Check sheet for the modelled part. Datum: model origin and axes. Units: mm. Coordinates: 2 decimals unless noted, no trailing zeros. Write each loop counter-clockwise with the first axis right and the second up, starting at its lowest first coordinate (ties: lowest second). Pieces come first, ordered by that corner, then holes. Notation, with made-up numbers: M -9,-14.5 L 40,-14.5 A27 ccw 40,4.5 Z; hole C 60.25,-13.75 d8. An arc over 180 degrees is marked long. Answer as CSV lines item,"result".
Autodesk Inventor part; units mm, degrees
ref_plane "YZ Plane" through (0, 0, 0) normal (1, 0, 0) x (0, 1, 0)
ref_plane "XZ Plane" through (0, 0, 0) normal (0, 1, 0) x (-1, 0, 0)
ref_plane "XY Plane" through (0, 0, 0) normal (0, 0, 1) x (1, 0, 0)
sketch "Sketch1" plane through (0, 0, 0) normal (0, 1, 0) x (-1, 0, 0)
  line L0 (-5, 10) -> (5, 10)
  line L1 (5, 10) -> (5, -10)
  line L2 (5, -10) -> (-5, -10)
  line L3 (-5, -10) -> (-5, 10)
  line L4 (-5, 10) -> (5, -10) construction
  line L5 (5, 10) -> (-5, -10) construction
  line L6 (12.5, 20) -> (-12.5, 20)
  line L7 (-12.5, 20) -> (-12.5, -110)
  line L8 (-12.5, -110) -> (12.5, -110)
  line L9 (12.5, -110) -> (12.5, 20)
  line L10 (1.59, -105) -> (-1.59, -105)
  line L11 (-1.59, -105) -> (-1.59, -90)
  line L12 (-1.59, -90) -> (1.59, -90)
  line L13 (1.59, -90) -> (1.59, -105)
  line L14 (1.59, -105) -> (-1.59, -90) construction
  line L15 (-1.59, -105) -> (1.59, -90) construction
  line L16 (7.5, -95.91) -> (-7.5, -95.91)
  line L17 (-7.5, -95.91) -> (-7.5, -99.09)
  line L18 (-7.5, -99.09) -> (7.5, -99.09)
  line L19 (7.5, -99.09) -> (7.5, -95.91)
  line L20 (7.5, -95.91) -> (-7.5, -99.09) construction
  line L21 (-7.5, -95.91) -> (7.5, -99.09) construction
  point P0 (0, 0)
  point P1 (0, 0)
  point P2 (0, 0)
  point P3 (0, -97.5)
  dimension "d24" = 10
  dimension "d25" = 20
  dimension "d26" = 25
  dimension "d27" = 130
  dimension "d28" = 20
  dimension "d29" = 12.5
  dimension "d37" = 3.18
  dimension "d38" = 15
  dimension "d39" = 15
  dimension "d40" = 3.18
  dimension "d41" = 12.5
  dimension "d42" = 12.5
extrude "Extrusion3" add sketch "Sketch1" along normal blind 3.18
properties part number "Brazo_Superior"
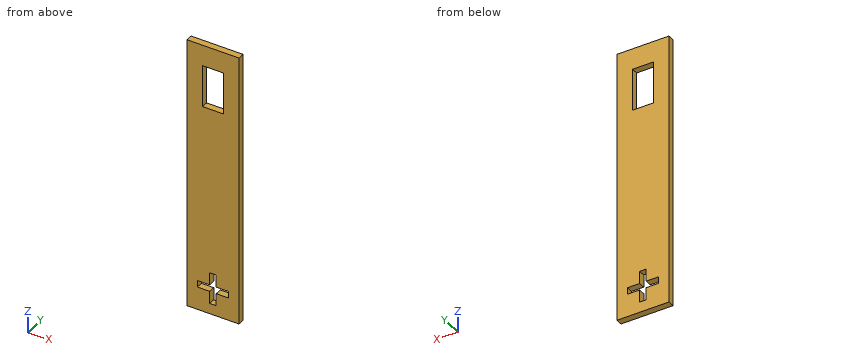
1) Section check B-B, the plane x = -0.25. Record the boundary of the cut face in (y, z), plus the area to 3 significant figures.
Answer key:
outline,"M 0,-110 L 3.18,-110 L 3.18,-105 L 0,-105 Z; M 0,-90 L 3.18,-90 L 3.18,-10 L 0,-10 Z; M 0,10 L 3.18,10 L 3.18,20 L 0,20 Z"
area,"302 mm2"
2) Section check A-A, the plane z = -97. Record the boundary of the cut face in (x, y).
Answer key:
outline,"M -12.5,0 L -7.5,0 L -7.5,3.18 L -12.5,3.18 Z; M 7.5,0 L 12.5,0 L 12.5,3.18 L 7.5,3.18 Z"
3) Section check C-C, the plane y = 0.75. Record the boundary of the cut face in (x, z), plus the area to 3 significant figures.
Answer key:
outline,"M -12.5,-110 L 12.5,-110 L 12.5,20 L -12.5,20 Z; hole M -7.5,-99.09 L -1.59,-99.09 L -1.59,-105 L 1.59,-105 L 1.59,-99.09 L 7.5,-99.09 L 7.5,-95.91 L 1.59,-95.91 L 1.59,-90 L -1.59,-90 L -1.59,-95.91 L -7.5,-95.91 Z; hole M -5,-10 L 5,-10 L 5,10 L -5,10 Z"
area,"2,960 mm2"
4) Thickness scan on line 1 along Z through (x, y) = (-4.5, 2.9); line 2 along Z through (x, y) = (-0.5, 0.4); line 3 along X through (y, z) = (1.75, -95.5). Record the ranges inside material, lowest first.
Answer key:
line 1,"z = -110 to -99.09, -95.91 to -10, 10 to 20"
line 2,"z = -110 to -105, -90 to -10, 10 to 20"
line 3,"x = -12.5 to -1.59, 1.59 to 12.5"
5) Section check D-D, the plane z = -3.5. Record the boundary of the cut face in (x, y), plus the area to 3 significant figures.
Answer key:
outline,"M -12.5,0 L -5,0 L -5,3.18 L -12.5,3.18 Z; M 5,0 L 12.5,0 L 12.5,3.18 L 5,3.18 Z"
area,"47.7 mm2"
6) Depth check by flat-ended pin: P1, Ø10, axis at x = 7, z = -67, coming from the -Y side. Enter the tip coordinate at first touch or a pass-through.
Answer key:
P1,"stops at y = 0"
